```python
from build123d import *

# Parameters (mm, degrees)
BOSS_EXTRUDE1_DEPTH = 58
CUT_EXTRUDE2_DEPTH  = 2
FILLET1_R           = 2


with BuildPart() as part:
    # Sketch1 → Boss-Extrude1 (new body)
    with BuildSketch(Plane(origin=(0, 0, 0), x_dir=(1, 0, 0), z_dir=(0, 1, 0))):
        with BuildLine():
            Line((-50, 16), (36, 16))
            Line((36, 16), (36, 14))
            Line((36, 14), (-50, 14))
            ThreePointArc((-50, 14), (-59.16515139, 10.583005244), (-63.856406461, 2))
            Line((-63.856406461, 2), (-64.928657629, 1.461225992))
            ThreePointArc((-64.928657629, 1.461225992), (-64.982153791, 0.731483276), (-65, 0))
            Line((-65, 0), (-66, 0))
            ThreePointArc((-66, 0), (-61.313708499, 11.313708499), (-50, 16))
        make_face()
    extrude(amount=BOSS_EXTRUDE1_DEPTH)

    # Sketch2 → Cut-Extrude2 (cut)
    with BuildSketch(Plane.XY.offset(-14)):
        Polygon((36, 58), (12.87566783, 58), (3.353954895, 58), (7.714660104, 38), (27.714660104, 38), (36, 0), align=None)
    extrude(amount=-CUT_EXTRUDE2_DEPTH, mode=Mode.SUBTRACT)

    # Fillet1
    fillet1_edges = [part.edges().sort_by_distance(p)[0] for p in [
        (36, 0, -15),
        (7.714660104, 38, -15),
        (3.353954895, 58, -15),
        (27.714660104, 38, -15),
    ]]
    fillet(fillet1_edges, radius=FILLET1_R)


solid = part.part
```
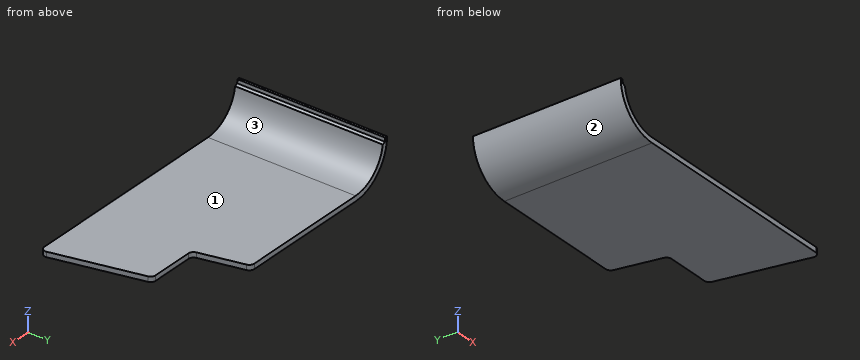
Work out the finished part from the listing and answer in its coordinate system (mm). Face numbers are marked on the shaded views. Round coordinates to 2 decimals unless told otherwise and drop trailing zeros. Write each loop counter-clockwise with the first axis right and the second up, starting at its lowest first coordinate (ties: lowest second). Pieces come first, ordered by that corner, then holes. Notation, with made-up numbers: (75.5, -5.5) -> (110.5, -5.5) arc R25 cw to (110.5, 29.5) -> close; hole circle Ø1 at (29, 15). An arc over 180 degrees is marked (long way). Write each question's results on one line, items separated by ' | '.
Q1. Section D-D, the plane y = 17.5 is taken. Write down the section's boundary in (x, z).
Data:
outline: (-66, 0) arc R16 ccw to (-50, -16) -> (32.18, -16) -> (32.18, -14) -> (-50, -14) arc R14 cw to (-63.86, -2) -> (-64.93, -1.46) arc R15 cw to (-65, 0) -> close
Q2. Flat-ended cylindrical pins translate along their axes: P1, Ø0.6, axis at x = 21, z = -14.5, coming from the +Y side; P2, Ø6, axis at y = 12, z = -4.5, coming from the +X side; P3, Ø12, axis at x = -34, y = 38, coming from the +Z side. Find the tip coordinate at first contact, or state that the pin passes through.
Data:
P1: y = 38 | P2: x = -61.82 | P3: z = -14
Q3. Section B-B, the plane x = 20 is taken. Write down the section's boundary in (y, z).
Data:
outline: (0, -16) -> (38, -16) -> (38, -14) -> (0, -14) -> close
Q4. Section C-C, the plane z = -7 is taken. Write down the section's boundary in (x, y), then the cut area to 3 significant figures.
Data:
outline: (-64.39, 0) -> (-62.12, 0) -> (-62.12, 58) -> (-64.39, 58) -> close | area: 131 mm^2
Q5. Section A-A, the plane y = 7.5 is taken. Write down the section's boundary in (x, z).
Data:
outline: (-66, 0) arc R16 ccw to (-50, -16) -> (34.36, -16) -> (34.36, -14) -> (-50, -14) arc R14 cw to (-63.86, -2) -> (-64.93, -1.46) arc R15 cw to (-65, 0) -> close
Q6. Determine the mould class of the marked faces 1, 2 and 3 for opening direction X: released by +X, released by -X, zero draft, split by the parting line, or undercut.
Data:
face 1: zero draft | face 2: released by -X | face 3: released by +X
Q7. Straight lines are drawn through the part: line 1 along Z through (x, y) = (-32, 3.5); line 2 along Y through (x, z) = (10.5, -14.25); line 3 along X through (y, z) = (14.5, -1.5). For each, find the intervals that lie inside material, in ascending order. Write a range as [from, to].
Data:
line 1: [-16, -14] | line 2: [0, 38] | line 3: [-65.93, -64.85]
